```python
from build123d import *

# Parameters (mm, degrees)
SM_BASE_FLANGE_2_DEPTH  = 10
HOLE_WIZARD_4_3_4_3_1_D = 4.3
HOLE_WIZARD_4_3_4_3_2_D = 4.3


# Sheet-metal steps are written as plain solids
with BuildPart() as part:
    # 草图18 → 基体-法兰2 (new body)
    with BuildSketch(Plane.XY):
        with BuildLine():
            Line((0, 20), (0, 3.7366))
            ThreePointArc((0, 3.7366), (1.094424801, 1.094424801), (3.7366, 0))
            Line((3.7366, 0), (20, 0))
            Line((20, 0), (20, 3))
            Line((20, 3), (3.7366, 3))
            ThreePointArc((3.7366, 3), (3.215745145, 3.215745145), (3, 3.7366))
            Line((3, 3.7366), (3, 20))
            Line((3, 20), (0, 20))
        make_face()
    extrude(amount=SM_BASE_FLANGE_2_DEPTH)

    # Ø4.3 (4.3) 直径孔1 (through all)
    with Locations(Plane.ZY):
        with Locations((5, 13)):
            Hole(HOLE_WIZARD_4_3_4_3_1_D / 2)

    # Ø4.3 (4.3) 直径孔2 (through all)
    with Locations(Plane(origin=(0, 0, 0), x_dir=(-1, 0, 0), z_dir=(0, -1, 0))):
        with Locations((-13, -5)):
            Hole(HOLE_WIZARD_4_3_4_3_2_D / 2)


solid = part.part
```
Work out the finished part from the listing and answer in its coordinate system (mm). A direction names the side the tool comes from. Coordinates: 2 decimals unless noted, no trailing zeros. Loops run counter-clockwise (first coordinate to the right, second up) from the corner with the lowest first, then second, coordinate; pieces in that order, holes last.
1) Section A-A (y = 13) is taken. Give the vertices of the cut face in (x, z).
Results:
outline: (0, 0) - (3, 0) - (3, 2.85) - (0, 2.85) - close; (0, 7.15) - (3, 7.15) - (3, 10) - (0, 10) - close
2) Consider probe 1 along Z at (x, y) = (13, 0.8); probe 2 along X at (y, z) = (17.5, 8); probe 3 along Y at (x, z) = (1, 3.5). Determine where each line is inside the solid, lowest interval first.
Results:
probe 1: z = 0 to 2.85, 7.15 to 10
probe 2: x = 0 to 3
probe 3: y = 1.19 to 11.46, 14.54 to 20
3) Flat-ended cylindrical pins translate along their axes: pin 1 (10 mm diameter, centred on x = 11, y = 8.5, fed in from -Z); pin 2 (3 mm diameter, centred on y = 16, z = 5.5, fed in from +X); pin 3 (3 mm diameter, centred on x = 14.5, z = 5.5, fed in from +Y). Find the tip coordinate at first contact, or state that the pin passes through.
Results:
pin 1: passes through
pin 2: stops at x = 3
pin 3: stops at y = 3
4) For a pull along Z with two mould halves and no side action, classify faces 3 (the flat face through (6.2, 2.6, 0)), 4 (the cylindrical face through (1.521, 11.692, 6.706)), 5 (the flat face through (2, 20, 5)) as +Z half, -Z half, draft (parallel to the pull), parting line (faces both ways), or undercut.
Results:
face 3: -Z half
face 4: undercut
face 5: draft
5) For faces 1 (the flat face through (3, 10, 5)), 2 (the flat face through (0, 10, 5)), determine the directions among +Z, -Z, +X, -X, +Y, -Y from which every point of the face is accessible in a straight line to the end or side of a thin tool.
Results:
face 1: +Z, -Z, +X, +Y
face 2: +Z, -Z, -X, +Y, -Y
6) Section D-D (z = 8.5) is taken. Give the vertices of the cut face in (x, y).
Results:
outline: (0, 3.74) arc R3.74 ccw to (3.74, 0) - (20, 0) - (20, 3) - (3.74, 3) arc R0.74 cw to (3, 3.74) - (3, 20) - (0, 20) - close
7) Section C-C (z = 6.25) is taken. Give the vertices of the cut face in (x, y), plus the area to 3 significant figures.
Results:
outline: (0, 3.74) arc R3.74 ccw to (3.74, 0) - (11.25, 0) - (11.25, 3) - (3.74, 3) arc R0.74 cw to (3, 3.74) - (3, 11.25) - (0, 11.25) - close; (0, 14.75) - (3, 14.75) - (3, 20) - (0, 20) - close; (14.75, 0) - (20, 0) - (20, 3) - (14.75, 3) - close
area: 87.1 mm2
